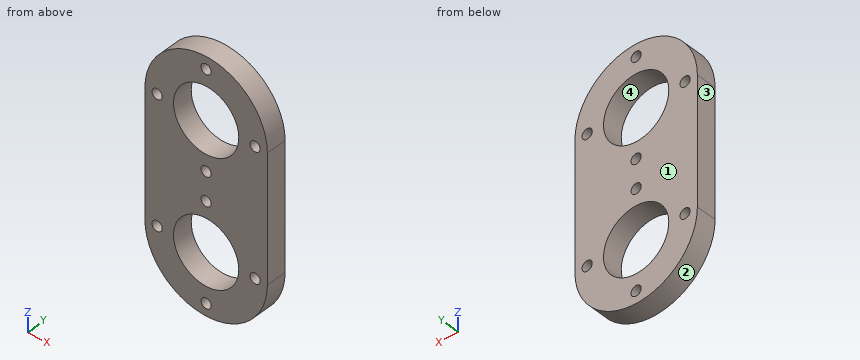
```python
from build123d import *

# Parameters (mm, degrees)
CROQUIS1_R              = 16
SALIENTE_EXTRUIR1_DEPTH = 10
SKETCH1_R               = 2.5
CUT_EXTRUDE1_DEPTH      = 69.709533545
CIRPATTERN1_COUNT       = 4
MIRROR1_COPY_1_SKETCH_R = 2.5
MIRROR1_COPY_1_DEPTH    = 69.709533545
MIRROR1_COPY_2_SKETCH_R = 2.5
MIRROR1_COPY_2_DEPTH    = 69.709533545
MIRROR1_COPY_3_SKETCH_R = 2.5
MIRROR1_COPY_3_DEPTH    = 69.709533545


with BuildPart() as part:
    # Croquis1 → Saliente-Extruir1 (new body)
    with BuildSketch(Plane(origin=(0, 0, 0), x_dir=(1, 0, 0), z_dir=(0, 1, 0))):
        with BuildLine():
            Line((30, 31), (30, -31))
            ThreePointArc((30, -31), (0, -61), (-30, -31))
            Line((-30, -31), (-30, 31))
            ThreePointArc((-30, 31), (0, 61), (30, 31))
        make_face()
        with Locations(Location((0, -31, 0), (0, 0, 270))):
            Circle(CROQUIS1_R, mode=Mode.SUBTRACT)
        with Locations(Location((0, 31, 0), (0, 0, 270))):
            Circle(CROQUIS1_R, mode=Mode.SUBTRACT)
    extrude(amount=SALIENTE_EXTRUIR1_DEPTH)

    # Sketch1 → Cut-Extrude1 (cut, through all)
    with BuildSketch(Plane(origin=(0, 10, 0), x_dir=(1, 0, 0), z_dir=(0, 1, 0))):
        with Locations(Location((24, 31, 0), (0, 0, 270))):
            Circle(SKETCH1_R)
    cut_extrude1 = extrude(amount=-CUT_EXTRUDE1_DEPTH, mode=Mode.SUBTRACT)

    # CirPattern1: Cut-Extrude1 ×4 about axis
    cirpattern1_axis = Axis((0, 0, -31), (0, 1, 0))
    for i in range(1, CIRPATTERN1_COUNT):
        add(cut_extrude1.rotate(cirpattern1_axis, i * 360 / CIRPATTERN1_COUNT), mode=Mode.SUBTRACT)

    # Mirror1: Cut-Extrude1 across plane
    add(cut_extrude1.mirror(Plane.XY), mode=Mode.SUBTRACT)

    # Mirror1 copy 1 sketch → Mirror1 copy 1 (cut, through all)
    with BuildSketch(Plane(origin=(31, 10, 31), x_dir=(0, 0, 1), z_dir=(0, 1, 0))):
        with Locations((24, -31)):
            Circle(MIRROR1_COPY_1_SKETCH_R)
    extrude(amount=-MIRROR1_COPY_1_DEPTH, mode=Mode.SUBTRACT)

    # Mirror1 copy 2 sketch → Mirror1 copy 2 (cut, through all)
    with BuildSketch(Plane(origin=(0, 10, 62), x_dir=(-1, 0, 0), z_dir=(0, 1, 0))):
        with Locations((24, -31)):
            Circle(MIRROR1_COPY_2_SKETCH_R)
    extrude(amount=-MIRROR1_COPY_2_DEPTH, mode=Mode.SUBTRACT)

    # Mirror1 copy 3 sketch → Mirror1 copy 3 (cut, through all)
    with BuildSketch(Plane(origin=(-31, 10, 31), x_dir=(0, 0, -1), z_dir=(0, 1, 0))):
        with Locations((24, -31)):
            Circle(MIRROR1_COPY_3_SKETCH_R)
    extrude(amount=-MIRROR1_COPY_3_DEPTH, mode=Mode.SUBTRACT)


solid = part.part
```
Geometry check sheet. Reference: the model listing, model coordinates, mm. Face numbers are marked on the shaded views. Coordinates: 2 decimals unless noted, no trailing zeros. Order: outer loops, then holes, each group sorted by start corner. A loop starts at its lowest first (then second) coordinate and runs counter-clockwise, first axis right, second up. Notation, with made-up numbers: (81, -25) - (126, -25) arc R18 ccw to (126, -16) - close; hole circle Ø4 at (23, -22.5). An arc over 180 degrees is marked (long way). Answer as a JSON object with one key per item and string values. Group by question number.
Item 1: Scan lines: probe 1 along X at (y, z) = (5.5, -31); probe 2 along Z at (x, y) = (26, 6); probe 3 along Z at (x, y) = (22, 4.25). Record each from-to range of solid material in increasing order.
Item 2: Sectioned sample at C-C, the plane y = 3. Give the number of separate pieces and of enclosed holes in the cut face, and give its area (3 significant figures).
Item 3: Sectioned sample at A-A, the plane x = -24. Record the cut outline in (y, z).
Item 4: Depth check by flat-ended pin: pin 1 Ø3 at (x, z) = (24, -31) entering from +Y; pin 2 Ø3 at (x, y) = (6.5, 3.5) entering from +Z; pin 3 Ø6 at (y, z) = (2, 45.5) entering from +X; pin 4 Ø6 at (x, y) = (-16, 8) entering from -Z. Enter the tip coordinate at first touch or a pass-through.
Item 5: Sectioned sample at D-D, the plane x = 0. Record the cut outline in (y, z), and give its area (3 significant figures).
Item 6: Sectioned sample at B-B, the plane z = -55. Record the cut outline in (x, y), and give its area (3 significant figures).
Item 7: Draft check along X on the marked faces 1, 2, 3 and 4. Enter one of: +X half, -X half, draft (parallel to the pull), parting line (faces both ways), or undercut.
Resolved:
{
 "1": {"probe 1": "-30 to -26.5, -21.5 to -16, 16 to 21.5, 26.5 to 30", "probe 2": "-45.97 to -32.5, -29.5 to 29.5, 32.5 to 45.97", "probe 3": "-51.4 to -32.5, -29.5 to 29.5, 32.5 to 51.4"},
 "2": {"separate pieces": "1", "enclosed holes": "10", "area": "4,780 mm^2"},
 "3": {"outline": "(0, -49) - (10, -49) - (10, -33.5) - (0, -33.5) - close; (0, -28.5) - (10, -28.5) - (10, 28.5) - (0, 28.5) - close; (0, 33.5) - (10, 33.5) - (10, 49) - (0, 49) - close"},
 "4": {"pin 1": "through", "pin 2": "z = 60.58", "pin 3": "x = 27.71", "pin 4": "z = -58.04"},
 "5": {"outline": "(0, -61) - (10, -61) - (10, -57.5) - (0, -57.5) - close; (0, -52.5) - (10, -52.5) - (10, -47) - (0, -47) - close; (0, -15) - (10, -15) - (10, -9.5) - (0, -9.5) - close; (0, -4.5) - (10, -4.5) - (10, 4.5) - (0, 4.5) - close; (0, 9.5) - (10, 9.5) - (10, 15) - (0, 15) - close; (0, 47) - (10, 47) - (10, 52.5) - (0, 52.5) - close; (0, 57.5) - (10, 57.5) - (10, 61) - (0, 61) - close", "area": "380 mm^2"},
 "6": {"outline": "(-18, 0) - (-2.5, 0) - (-2.5, 10) - (-18, 10) - close; (2.5, 0) - (18, 0) - (18, 10) - (2.5, 10) - close", "area": "310 mm^2"},
 "7": {"face 1": "draft", "face 2": "parting line", "face 3": "-X half", "face 4": "undercut"}
}
